```python
from build123d import *

# Parameters (mm, degrees)
SKETCH1_W           = 60
SKETCH1_H           = 15
BOSS_EXTRUDE1_DEPTH = 3
BOSS_EXTRUDE2_DEPTH = 6
CUT_EXTRUDE1_DEPTH  = 34.972930401
SKETCH5_W           = 60
SKETCH5_H           = 1.5
BOSS_EXTRUDE3_DEPTH = 10


with BuildPart() as part:
    # Sketch1 → Boss-Extrude1 (new body)
    with BuildSketch(Plane.XY):
        Rectangle(SKETCH1_W, SKETCH1_H)
    extrude(amount=BOSS_EXTRUDE1_DEPTH)

    # Sketch3 → Boss-Extrude2 (add)
    with BuildSketch(Plane(origin=(0, -2.5, 0), x_dir=(-1, 0, 0), z_dir=(0, -1, 0))):
        Polygon((-14.5, 0), (-17.5, 0), (-17.5, 3.4), (-18.9, 3.4), (-18.9, 5.4), (-13.1, 5.4), (-13.1, 3.4), (-14.5, 3.4), align=None)
        Polygon((14.5, 3.4), (14.5, 0), (17.5, 0), (17.5, 3.4), (18.9, 3.4), (18.9, 5.4), (13.1, 5.4), (13.1, 3.4), align=None)
    extrude(amount=-BOSS_EXTRUDE2_DEPTH)

    # Sketch4 → Cut-Extrude1 (cut, through all)
    with BuildSketch(Plane(origin=(0, 7.5, 0), x_dir=(1, 0, 0), z_dir=(0, 1, 0))):
        Polygon((30, 0), (22, 0), (23.5, -1.5), (30, -1.5), align=None)
        Polygon((0, 0), (0, -1.5), (8.5, -1.5), (10, 0), align=None)
    cut_extrude1 = extrude(amount=-CUT_EXTRUDE1_DEPTH, mode=Mode.SUBTRACT)

    # Mirror1: Cut-Extrude1 across plane
    add(cut_extrude1.mirror(Plane(origin=(0, 0, 0), x_dir=(0, 0, 1), z_dir=(1, 0, 0))), mode=Mode.SUBTRACT)

    # Sketch5 → Boss-Extrude3 (add)
    with BuildSketch(Plane(origin=(0, 7.5, 0), x_dir=(1, 0, 0), z_dir=(0, 1, 0))):
        with Locations((0, -2.25)):
            Rectangle(SKETCH5_W, SKETCH5_H)
    boss_extrude3 = extrude(amount=BOSS_EXTRUDE3_DEPTH)

    # Mirror2: Boss-Extrude3 across plane
    add(boss_extrude3.mirror(Plane.ZX))


solid = part.part
```
Input: part model. Units: mm. Frame: model coordinates. A direction names the side the tool comes from. Round coordinates to 2 decimals unless told otherwise and drop trailing zeros. Order: outer loops, then holes, each group sorted by start corner. A loop starts at its lowest first (then second) coordinate and runs counter-clockwise, first axis right, second up. Notation, with made-up numbers: (-19.75, 56) - (-11.75, 56) arc R37 cw to (-11.75, 92) - close; hole circle Ø6 at (7, 48.5). An arc over 180 degrees is marked (long way). Answer in a Markdown table with one row per item.
Item 1: Section query A-A (z = -2.5). Return the cut outline in (x, y), then the cut area to 3 significant figures.
Model answer:
| item | result |
|---|---|
| outline | (-17.5, -2.5) - (-14.5, -2.5) - (-14.5, 3.5) - (-17.5, 3.5) - close; (14.5, -2.5) - (17.5, -2.5) - (17.5, 3.5) - (14.5, 3.5) - close |
| area | 36.0 mm² |
Item 2: Pin query (flat end, axial travel): pin 1 (2 mm diameter, centred on y = 0, z = -4.5, fed in from -X); pin 2 (1 mm diameter, centred on y = 0, z = -2, fed in from +X); pin 3 (1.6 mm diameter, centred on x = 17, z = -2, fed in from +Y); pin 4 (2 mm diameter, centred on y = 14, z = 0, fed in from +X). Return the tip coordinate at first contact, or that it passes through.
Model answer:
| item | result |
|---|---|
| pin 1 | stops at x = -18.9 |
| pin 2 | stops at x = 17.5 |
| pin 3 | stops at y = 3.5 |
| pin 4 | passes through |
Item 3: Section query C-C (x = -16.5). Return the cut outline in (y, z), then the cut area to 3 significant figures.
Model answer:
| item | result |
|---|---|
| outline | (-17.5, 1.5) - (-7.5, 1.5) - (-7.5, 0) - (-2.5, 0) - (-2.5, -5.4) - (3.5, -5.4) - (3.5, 0) - (7.5, 0) - (7.5, 1.5) - (17.5, 1.5) - (17.5, 3) - (-17.5, 3) - close |
| area | 107 mm² |
Item 4: Section query B-B (y = -1.5). Return the cut outline in (x, z).
Model answer:
| item | result |
|---|---|
| outline | (-30, 1.5) - (-23.5, 1.5) - (-22, 0) - (-17.5, 0) - (-17.5, -3.4) - (-18.9, -3.4) - (-18.9, -5.4) - (-13.1, -5.4) - (-13.1, -3.4) - (-14.5, -3.4) - (-14.5, 0) - (-10, 0) - (-8.5, 1.5) - (8.5, 1.5) - (10, 0) - (14.5, 0) - (14.5, -3.4) - (13.1, -3.4) - (13.1, -5.4) - (18.9, -5.4) - (18.9, -3.4) - (17.5, -3.4) - (17.5, 0) - (22, 0) - (23.5, 1.5) - (30, 1.5) - (30, 3) - (-30, 3) - close |
Item 5: Section query D-D (y = -5). Return the cut outline in (x, z), then the cut area to 4 significant figures.
Model answer:
| item | result |
|---|---|
| outline | (-30, 1.5) - (-23.5, 1.5) - (-22, 0) - (-10, 0) - (-8.5, 1.5) - (8.5, 1.5) - (10, 0) - (22, 0) - (23.5, 1.5) - (30, 1.5) - (30, 3) - (-30, 3) - close |
| area | 130.5 mm² |
Item 6: Line query: line 1 (Z direction, x = 20, y = -11.5); line 2 (Z direction, x = -15.5, y = -4.5); line 3 (X direction, y = -6, z = 1). Output: solid intervals per line, ascending.
Model answer:
| item | result |
|---|---|
| line 1 | z = 1.5 to 3 |
| line 2 | z = 0 to 3 |
| line 3 | x = -23 to -9, 9 to 23 |
Item 7: Reachability of faces 4 (the flat face through (0, 0, 1.5)), 5 (the flat face through (-16, 7.5, 1)), 6 (the flat face through (17.5, 0, -2)) from +Z, -Z, +X, -X, +Y, -Y: full face, straight path, thin tool, end or side. Return the list, or none.
Model answer:
| item | result |
|---|---|
| face 4 | -Z |
| face 5 | -Z, +X, -X, +Y |
| face 6 | +X, +Y, -Y |
Item 8: Mould query, pull axis Z, two halves, no side actions, for faces 1 (the flat face through (9, 0, 1)), 2 (the flat face through (-13.1, 0, -4)), 3 (the flat face through (18, 0, -3.4)). Classes: released by +Z, released by -Z, zero draft, split by the parting line, or undercut.
Model answer:
| item | result |
|---|---|
| face 1 | released by -Z |
| face 2 | zero draft |
| face 3 | undercut |
